Build history of the part. All positions in model axes, mm. A direction names the side the tool comes from. Give positions to 0.01 mm unless a question says otherwise; leave off trailing zeros. Loops run counter-clockwise (first coordinate to the right, second up) from the corner with the lowest first, then second, coordinate; pieces in that order, holes last.
1) Band-saw the part on A-A on x = 7. List the corners of the cut face in (y, z).
2) Flat gauge pins, fed straight in: P1, Ø7.5, axis at x = 5.5, z = -21, coming from the -Y side; P2, Ø12, axis at x = -15, y = 84.5, coming from the -Z side. Where does each tip first touch, or does it go through?
3) 3-axis set-ups, long thin cutter, end or side, ignore diameter. For faces 1 (the flat face through (0, 50, -30)), 2 (the flat face through (-20, 59, -30)), 3 (the cylindrical face through (10.807, 114.664, -62.465)): which of +Z, -Z, +X, -X, +Y, -Y reach the whole face in a straight line?
4) Wall check: line 1 (Y direction, x = 1, z = -33); line 2 (Z direction, x = -17, y = 41); line 3 (X direction, y = 77.5, z = -6). Give the ranges that are in metal, low to high.
5) Band-saw the part on C-C on z = -14. List the corners of the cut face in (x, y), then the cut area to 3 significant figures.
6) Band-saw the part on B-B on y = 104.5. List the corners of the cut face in (x, z).
7) Band-saw the part on D-D on x = -13.5. List the corners of the cut face in (y, z).
```python
from build123d import *

# Parameters (mm, degrees)
SKETCH1_W           = 20
SKETCH1_H           = 60
BOSS_EXTRUDE1_DEPTH = 120
SKETCH2_W           = 60
SKETCH2_H           = 17.921787448
BOSS_EXTRUDE2_DEPTH = 15
SKETCH3_R           = 4.625
BOSS_EXTRUDE3_DEPTH = 5


with BuildPart() as part:
    # Sketch1 → Boss-Extrude1 (new body)
    with BuildSketch(Plane(origin=(0, 0, 0), x_dir=(1, 0, 0), z_dir=(0, 1, 0))):
        with Locations((-10, 30)):
            Rectangle(SKETCH1_W, SKETCH1_H)
    extrude(amount=BOSS_EXTRUDE1_DEPTH)

    # Sketch2 → Boss-Extrude2 (add)
    with BuildSketch(Plane(origin=(0, 0, 0), x_dir=(0, 0, -1), z_dir=(1, 0, 0))):
        with Locations((30, 111.039106276)):
            Rectangle(SKETCH2_W, SKETCH2_H)
    extrude(amount=BOSS_EXTRUDE2_DEPTH)

    # Sketch3 → Boss-Extrude3 (add)
    with BuildSketch(Plane(origin=(0, 0, -60), x_dir=(-1, 0, 0), z_dir=(0, 0, -1))):
        with Locations(Location((-8.672680841, 110.56115287, 0), (0, 0, 180))):
            Circle(SKETCH3_R)
    extrude(amount=BOSS_EXTRUDE3_DEPTH)


solid = part.part
```
Findings below:
1. outline: (102.08, -60) - (106.25, -60) - (106.25, -65) - (114.87, -65) - (114.87, -60) - (120, -60) - (120, 0) - (102.08, 0) - close
2. P1: stops at y = 102.08
2. P2: stops at z = -60
3. face 1: +Z, -Z, +X, -Y
3. face 2: +Z, -Z, -X, +Y, -Y
3. face 3: -Z
4. line 1: y = 102.08 to 120
4. line 2: z = -60 to 0
4. line 3: x = -20 to 0
5. outline: (-20, 0) - (0, 0) - (0, 102.08) - (15, 102.08) - (15, 120) - (-20, 120) - close
5. area: 2,670 mm2
6. outline: (-20, -60) - (15, -60) - (15, 0) - (-20, 0) - close
7. outline: (0, -60) - (120, -60) - (120, 0) - (0, 0) - close
